Autodesk Inventor part; units mm, degrees
ref_plane "YZ Plane" through (0, 0, 0) normal (1, 0, 0) x (0, 1, 0)
ref_plane "XZ Plane" through (0, 0, 0) normal (0, 1, 0) x (-1, 0, 0)
ref_plane "XY Plane" through (0, 0, 0) normal (0, 0, 1) x (1, 0, 0)
sketch "Эскиз1" plane through (0, 0, 0) normal (0, 0, 1) x (1, 0, 0)
  line L0 (-7, -3.5) -> (7, -3.5) construction
  line L1 (7, -3.5) -> (7, 3.5)
  line L2 (7, 3.5) -> (-7, 3.5)
  line L3 (-7, 3.5) -> (-7, -3.5)
  line L4 (-7, -3.5) -> (7, 3.5) construction
  line L5 (7, -3.5) -> (-7, 3.5) construction
  line L6 (0, -3.5) -> (0, -12.5) construction
  line L7 (-7, -3.5) -> (-3.289, -13.697)
  line L8 (7, -3.5) -> (3.289, -13.697)
  arc A0 (-3.289, -13.697) -> (3.289, -13.697) centre (0, -12.5) ccw
  point P0 (0, 0)
  point P1 (0, 0)
  point P2 (0, 0)
  point P3 (0, 0)
  dimension "d0" = 14
  dimension "d1" = 7
  dimension "d4" = 9
  dimension "d5" = 3.5
extrude "Выдавливание1" add sketch "Эскиз1" along normal blind 1.5
sketch "Эскиз4" plane through (0, 0, 1.5) normal (0, 0, 1) x (1, 0, 0)
  line L0 (7, 3.5) -> (-7, 3.5)
  line L1 (7, -3.5) -> (7, 3.5)
  line L2 (-7, 3.5) -> (-7, -3.5)
  line L3 (-7, -3.5) -> (7, -3.5)
  point P0 (0, 0)
extrude "Выдавливание6" add sketch "Эскиз4" along normal blind 3.6
sketch "Эскиз2" plane through (0, 0, 1.5) normal (0, 0, 1) x (1, 0, 0)
  arc A0 (-3.289, -13.697) -> (3.289, -13.697) centre (0, -12.5) ccw construction
  circle A1 centre (0, -12.5) radius 1.25
  point P0 (0, 0)
  dimension "d8" = 2.5
extrude "Выдавливание9" add sketch "Эскиз2" along normal blind 5
fillet "Сопряжение1" radius 3.5 2 edges at (7, 3.5, 2.55) (-7, 3.5, 2.55)
sketch "Эскиз5" plane through (0, 0, 5.1) normal (0, 0, 1) x (1, 0, 0)
  circle A0 centre (0, -9.5) radius 1.5 construction
  line L0 (7, -3.5) -> (-7, -3.5) construction
  line L1 (0, -3.5) -> (0, 3.5) construction
  line L2 (-7, 3.5) -> (7, 3.5) construction
  circle A1 centre (3.5, 0) radius 0.5
  line L3 (3.5, 3.5) -> (3.5, 0) construction
  line L4 (3.5, 0) -> (0, 0) construction
  circle A2 centre (-3.5, 0) radius 0.5
  dimension "d34" = 1
hole "Отверстие1" at (-3.5, 0, 5.1) at (3.5, 0, 5.1) direction (0, 0, -1) diameter 1 end through all countersink diameter 1.5 countersink angle 90
properties part number "переходник"
Could you check a few things on this model? Use its own coordinates, in mm. A direction names the side the tool comes from. Give positions to 0.01 mm unless a question says otherwise; leave off trailing zeros. Order: outer loops, then holes, each group sorted by start corner. A loop starts at its lowest first (then second) coordinate and runs counter-clockwise, first axis right, second up. Notation, with made-up numbers: (82, 70) - (105, 70) arc R20 ccw to (105, 75) - close; hole circle Ø9 at (70, 29.5). An arc over 180 degrees is marked (long way). One line per item, written item: value. Start each with the question number.
1. If I drill on probe 1 along X at (y, z) = (0, 2.2); probe 2 along Y at (x, z) = (3.5, 2.55); probe 3 along Z at (x, y) = (4, 2.25), over which ranges is the centre line in solid material (lowest first)?
2. For P1, Ø7.5, axis at x = -2, y = 1.5, coming from the +Z side; P2, Ø1.8, axis at x = -1.5, z = 2.5, coming from the -Y side, each with a flat end and sliding along its axis, tell me the tip position at first contact or that it passes through.
3. For faces 1 (the face through (-7, -2, 3)), 2 (the face through (0, 0, 5.1)), which set-ups out of +Z, -Z, +X, -X, +Y, -Y let a thin tool reach every point of the face, with its end or its side?
4. Imagine slicing it at A-A on z = 2.75. List the corners of the cut face in (x, y) for me.
5. Thinking about a two-plate mould opening in X: for faces 3 (the face through (-4, 0, 2)), 4 (the face through (0, -3.5, 3)), 5 (the face through (-0.16, -13.74, 3.96)), which applies, +X half, -X half, draft (parallel to the pull), parting line (faces both ways), or undercut?
6. Imagine slicing it at D-D on y = -0.25. Give the number of separate pieces and of enclosed holes in the cut face, plus the area to 3 significant figures.
7. Imagine slicing it at C-C on y = -12.5. List the corners of the cut face in (x, z) for me, plus the area to 3 significant figures.
8. Imagine slicing it at B-B on x = 0. List the corners of the cut face in (y, z) for me, plus the area to 4 significant figures.
Values:
1. probe 1: -7 to -4, -3 to 3, 4 to 7
1. probe 2: -3.5 to -0.5, 0.5 to 3.5
1. probe 3: 0 to 5.1
2. P1: z = 5.1
2. P2: y = -13.6
3. face 1: +Z, -Z, -X, +Y, -Y
3. face 2: +Z, +X, -X, +Y
4. outline: (-7, -3.5) - (7, -3.5) - (7, 0) arc R3.5 ccw to (3.5, 3.5) - (-3.5, 3.5) arc R3.5 ccw to (-7, 0) - close; circle Ø2.5 at (0, -12.5); hole circle Ø1 at (-3.5, 0); hole circle Ø1 at (3.5, 0)
5. face 3: undercut
5. face 4: draft
5. face 5: parting line
6. separate pieces: 3
6. enclosed holes: 0
6. area: 62.4 mm²
7. outline: (-3.72, 0) - (3.72, 0) - (3.72, 1.5) - (1.25, 1.5) - (1.25, 6.5) - (-1.25, 6.5) - (-1.25, 1.5) - (-3.72, 1.5) - close
7. area: 23.7 mm²
8. outline: (-16, 0) - (3.5, 0) - (3.5, 5.1) - (-3.5, 5.1) - (-3.5, 1.5) - (-11.25, 1.5) - (-11.25, 6.5) - (-13.75, 6.5) - (-13.75, 1.5) - (-16, 1.5) - close
8. area: 66.95 mm²
